Check sheet for the modelled part. Datum: model origin and axes. Units: mm. Face numbers are marked on the shaded views. A direction names the side the tool comes from. Round coordinates to 2 decimals unless told otherwise and drop trailing zeros. Order: outer loops, then holes, each group sorted by start corner. A loop starts at its lowest first (then second) coordinate and runs counter-clockwise, first axis right, second up.
Q1. Set-up check for the marked faces 5, 6, 7 and 8: record each of +Z, -Z, +X, -X, +Y, -Y from which the full face is reachable in a straight line by a thin tool's end or side.
Q2. Mould release check, pull along Y, two halves, no side actions. Record for the marked faces 1, 2, 3 and 4: +Y half, -Y half, draft (parallel to the pull), parting line (faces both ways), or undercut.
Q3. Cross-section at D-D on z = -14. Record the cut outline in (x, y).
Q4. Scan lines: probe 1 along Y at (x, z) = (0, 3); probe 2 along Z at (x, y) = (-4, 4); probe 3 along Y at (x, z) = (4.5, -13). Record each from-to range of solid material in increasing order.
Q5. Cross-section at A-A on y = 0. Give the number of separate pieces and of enclosed holes in the cut face, then the cut area to 3 significant figures.
Q6. Depth check by flat-ended pin: P1, Ø2.5, axis at x = 0, y = -19.69, coming from the +Z side; P2, Ø16.5, axis at y = 2.5, z = -19.5, coming from the -X side; P3, Ø10, axis at y = -21.5, z = -0.5, coming from the +X side; P4, Ø6, axis at y = 7, z = -12, coming from the +X side. Enter the tip coordinate at first touch or a pass-through.
Q7. Cross-section at B-B on x = -8.5. Record the cut outline in (y, z), then the cut area to 3 significant figures.
from build123d import *

# Parameters (mm, degrees)
SKETCH1_R                                       = 29.692527183
SKETCH1_R_2                                     = 22.692527183
SKETCH1_R_3                                     = 19.692527183
SKETCH1_R_4                                     = 16.692527183
BOSS_EXTRUDE1_DEPTH                             = 5
SKETCH9_W                                       = 27.5
SKETCH9_H                                       = 28
BOSS_EXTRUDE2_DEPTH                             = 7.5
SKETCH10_W                                      = 23.5
SKETCH10_H                                      = 25.45
CUT_EXTRUDE1_DEPTH                              = 6.1
SKETCH12_W                                      = 12
SKETCH12_H                                      = 11
CUT_EXTRUDE2_DEPTH                              = 3
CUT_EXTRUDE3_REACH                              = 55.407
SKETCH11_W                                      = 9.585282086
SKETCH11_H                                      = 9.717675131
CSK_FOR_M3_FLAT_HEAD_MACHINE_SCREW1_D           = 3.4
CSK_FOR_M3_FLAT_HEAD_MACHINE_SCREW1_DEPTH       = 12
CSK_FOR_M3_FLAT_HEAD_MACHINE_SCREW1_CSINK_D     = 7.3
CSK_FOR_M3_FLAT_HEAD_MACHINE_SCREW1_CSINK_ANGLE = 90
CSK_FOR_M3_FLAT_HEAD_MACHINE_SCREW1_TIP         = 1.021463052


with BuildPart() as part:
    # Sketch1 → Boss-Extrude1 (new body)
    # profile 1 of 4: a face of its own
    with BuildSketch(Plane(origin=(0, 0, 0), x_dir=(-1, 0, 0), z_dir=(0, 0, 1))):
        with Locations(Location((0, 0, 0), (0, 0, 180))):
            Circle(SKETCH1_R)
        Circle(SKETCH1_R_2, mode=Mode.SUBTRACT)
    # profile 2 of 4: a face of its own
    with BuildSketch(Plane(origin=(0, 0, 0), x_dir=(-1, 0, 0), z_dir=(0, 0, 1))):
        Circle(SKETCH1_R_2)
        Circle(SKETCH1_R_3, mode=Mode.SUBTRACT)
    # profile 3 of 4: a face of its own
    with BuildSketch(Plane(origin=(0, 0, 0), x_dir=(-1, 0, 0), z_dir=(0, 0, 1))):
        Circle(SKETCH1_R_3)
        Circle(SKETCH1_R_4, mode=Mode.SUBTRACT)
    # profile 4 of 4: a face of its own
    with BuildSketch(Plane(origin=(0, 0, 0), x_dir=(-1, 0, 0), z_dir=(0, 0, 1))):
        with BuildLine():
            Line((14.058465911, 9), (-14.058465911, 9))
            ThreePointArc((-14.058465911, 9), (-16.692527183, 0), (-14.058465911, -9))
            Line((-14.058465911, -9), (14.058465911, -9))
            ThreePointArc((14.058465911, -9), (16.020483578, -4.688770595), (16.692527183, 0))
            ThreePointArc((16.692527183, 0), (16.020483578, 4.688770595), (14.058465911, 9))
        make_face()
    extrude(amount=BOSS_EXTRUDE1_DEPTH)

    # Sketch9 → Boss-Extrude2 (add, symmetric)
    with BuildSketch(Plane(origin=(0, 0, 0), x_dir=(1, 0, 0), z_dir=(0, 1, 0))):
        with Locations((0, 14)):
            Rectangle(SKETCH9_W, SKETCH9_H)
    extrude(amount=BOSS_EXTRUDE2_DEPTH, both=True)

    # Sketch10 → Cut-Extrude1 (cut, symmetric)
    with BuildSketch(Plane(origin=(0, 0, 0), x_dir=(1, 0, 0), z_dir=(0, 1, 0))):
        with Locations((0, 12.775)):
            Rectangle(SKETCH10_W, SKETCH10_H)
    extrude(amount=CUT_EXTRUDE1_DEPTH, both=True, mode=Mode.SUBTRACT)

    # Sketch12 → Cut-Extrude2 (cut)
    with BuildSketch(Plane.XY.offset(-28)):
        with Locations((3.75, 0)):
            Rectangle(SKETCH12_W, SKETCH12_H)
    extrude(amount=CUT_EXTRUDE2_DEPTH, mode=Mode.SUBTRACT)

    # Cut-Extrude3: up to this face of the body (flat: up to its plane)
    cut_extrude3_end = Plane(part.part.faces().sort_by_distance((0, 0, -0.05))[0])
    # Sketch11 → Cut-Extrude3 (cut, up to the picked face)
    with BuildSketch(Plane.XY.offset(5), mode=Mode.PRIVATE) as cut_extrude3_sk1:
        with Locations((8.957358957, -0.433824782)):
            Rectangle(SKETCH11_W, SKETCH11_H)
    cut_extrude3_tool1 = split(extrude(cut_extrude3_sk1.sketch, amount=-CUT_EXTRUDE3_REACH, mode=Mode.PRIVATE), bisect_by=cut_extrude3_end, keep=Keep.BOTH, mode=Mode.PRIVATE)
    add(cut_extrude3_tool1.solids().sort_by(Axis((8.957359, -0.433825, 5), (0, 0, -1)))[0], mode=Mode.SUBTRACT)

    # CSK for M3 Flat Head Machine Screw1
    with Locations(Plane(origin=(0, 0, 0), x_dir=(1, 0, 0), z_dir=(0, 0, -1))):
        with Locations((-19.692527183, 0), (0, 19.692527183), (0, -19.692527183), (19.692527183, 0)):
            CounterSinkHole(CSK_FOR_M3_FLAT_HEAD_MACHINE_SCREW1_D / 2, CSK_FOR_M3_FLAT_HEAD_MACHINE_SCREW1_CSINK_D / 2, depth=CSK_FOR_M3_FLAT_HEAD_MACHINE_SCREW1_DEPTH, counter_sink_angle=CSK_FOR_M3_FLAT_HEAD_MACHINE_SCREW1_CSINK_ANGLE)
            with Locations((0, 0, -(CSK_FOR_M3_FLAT_HEAD_MACHINE_SCREW1_DEPTH + CSK_FOR_M3_FLAT_HEAD_MACHINE_SCREW1_TIP / 2))):  # 118° drill point
                Cone(0, CSK_FOR_M3_FLAT_HEAD_MACHINE_SCREW1_D / 2, CSK_FOR_M3_FLAT_HEAD_MACHINE_SCREW1_TIP, mode=Mode.SUBTRACT)


solid = part.part
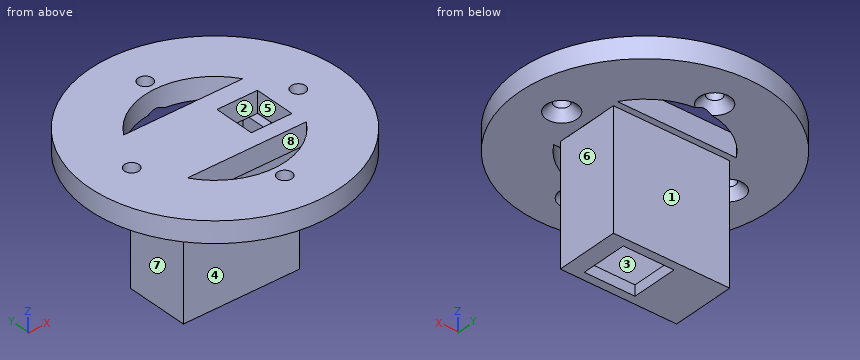
Results found:
1. face 5: +Z
1. face 6: -Z, +X, +Y, -Y
1. face 7: -Z, -X, +Y, -Y
1. face 8: +Z, -Z
2. face 1: +Y half
2. face 2: undercut
2. face 3: undercut
2. face 4: -Y half
3. outline: (-13.75, -7.5) - (13.75, -7.5) - (13.75, 7.5) - (-13.75, 7.5) - close; hole (-11.75, -6.1) - (11.75, -6.1) - (11.75, 6.1) - (-11.75, 6.1) - close
4. probe 1: y = -29.69 to -21.39, -17.99 to -16.69, -9 to 9, 16.69 to 17.99, 21.39 to 29.69
4. probe 2: z = -28 to -25.5, -0.05 to 5
4. probe 3: y = -7.5 to -6.1, 6.1 to 7.5
5. separate pieces: 5
5. enclosed holes: 0
5. area: 349 mm2
6. P1: passes through
6. P2: stops at x = -13.75
6. P3: stops at x = 24.67
6. P4: stops at x = 13.75
7. outline: (-28.45, 0) - (-14.37, 0) - (-14.37, 5) - (-28.45, 5) - close; (-9, 0) - (-7.5, 0) - (-7.5, -28) - (7.5, -28) - (7.5, 0) - (9, 0) - (9, 5) - (-9, 5) - close; (14.37, 0) - (28.45, 0) - (28.45, 5) - (14.37, 5) - close; hole (-6.1, -25.5) - (6.1, -25.5) - (6.1, -0.05) - (-6.1, -0.05) - close
7. area: 340 mm2
